from build123d import *

# Parameters (mm, degrees)
F1_ANGLE_BACK  = 30
F1_ANGLE       = 120
F2_R           = 2
F4_DEPTH       = 25
F4_DEPTH_BACK  = 25
F5_DEPTH       = 25
F5_DEPTH_BACK  = 25
F8_R           = 5
F10_DEPTH      = 33.4248144675
F10_DEPTH_BACK = 33.4248144675
F12_DEPTH      = 50
F12_DEPTH_BACK = 50


# Not quite as in the source:
# - after a boolean that leaves OpenCascade's solid faulty, fix() repairs it
# - a feature of the source that left no trace in its solid (it failed there, or was rolled back) is left out


with BuildPart() as f1:
    # F0 (on Top) → F1 (revolve)
    with BuildSketch(Plane.XY, mode=Mode.PRIVATE) as f1_sk:
        with BuildLine():
            Line((9.6206148389, -1.9516889929), (7.6821408379, -2.0284350604))
            Line((7.6821408379, -2.0284350604), (30.2427770644, -88.5876107865))
            ThreePointArc((30.2427770644, -88.5876107865), (29.2549191731, -93.4242240292), (24.8238143675, -95.6))
            Line((24.8238143675, -95.6), (-24.8238143675, -95.6))
            ThreePointArc((-24.8238143675, -95.6), (-29.2549191731, -93.4242240292), (-30.2427770644, -88.5876107865))
            Line((-30.2427770644, -88.5876107865), (-7.6821408379, -2.0284350604))
            Line((-7.6821408379, -2.0284350604), (-9.6206148389, -1.9516889929))
            Line((-9.6206148389, -1.9516889929), (-13.35, -1.9516889929))
            Line((-13.35, -1.9516889929), (-13.35, 37))
            Line((-13.35, 37), (-16.35, 37))
            Line((-16.35, 37), (-16.35, -4.9516889929))
            Line((-16.35, -4.9516889929), (-11.5442770978, -4.9516889929))
            Line((-11.5442770978, -4.9516889929), (-33.1457927948, -87.8309737078))
            ThreePointArc((-33.1457927948, -87.8309737078), (-31.6287253189, -95.2586297591), (-24.8238143675, -98.6))
            Line((-24.8238143675, -98.6), (24.8238143675, -98.6))
            ThreePointArc((24.8238143675, -98.6), (31.6287253189, -95.2586297591), (33.1457927948, -87.8309737078))
            Line((33.1457927948, -87.8309737078), (11.5442770978, -4.9516889929))
            Line((11.5442770978, -4.9516889929), (16.35, -4.9516889929))
            Line((16.35, -4.9516889929), (16.35, 37))
            Line((16.35, 37), (13.35, 37))
            Line((13.35, 37), (13.35, -1.9516889929))
            Line((13.35, -1.9516889929), (9.6206148389, -1.9516889929))
        make_face()
    revolve(f1_sk.sketch.rotate(Axis((0.7210588083, 37, 0), (1, 0, 0)), -F1_ANGLE_BACK), axis=Axis((0.7210588083, 37, 0), (1, 0, 0)), revolution_arc=F1_ANGLE)

    # F2
    f2_edges = [f1.edges().sort_by_distance(p)[0] for p in [
        (7.682141, 3.200384, -19.514218),
        (11.544277, 0.668772, -20.975844),
        (16.35, 0.668772, -20.975844),
        (-7.682141, 3.200384, -19.514218),
        (-16.35, 0.668772, -20.975844),
        (-11.544277, 0.668772, -20.975844),
    ]]
    fillet(f2_edges, radius=F2_R)

    # F3 (on Right) → F4 (join, two sides)
    with BuildSketch(Plane.YZ) as f4_sk:
        with BuildLine():
            Line((51.55, 6), (26.6076951546, 6))
            Line((26.6076951546, 6), (34.6184301396, 1.375))
            ThreePointArc((34.6184301396, 1.375), (37.711752374, 2.6562960223), (39.75, 0))
            ThreePointArc((39.75, 0), (38.9445436483, -1.9445436483), (37, -2.75))
            Line((37, -2.75), (37, -6))
            Line((37, -6), (51.55, -6))
            Line((51.55, -6), (51.55, 6))
        make_face()
        with BuildLine():
            ThreePointArc((47.3738633754, 0.95), (47.505593785, 0.4830952573), (47.55, 0))
            ThreePointArc((47.55, 0), (47.505593785, -0.4830952573), (47.3738633754, -0.95))
            ThreePointArc((47.3738633754, -0.95), (46.7738329701, -1.8738329701), (45.85, -2.4738633754))
            ThreePointArc((45.85, -2.4738633754), (44.9, -2.65), (43.95, -2.4738633754))
            ThreePointArc((43.95, -2.4738633754), (43.0261670299, -1.8738329701), (42.4261366246, -0.95))
            ThreePointArc((42.4261366246, -0.95), (42.25, 0), (42.4261366246, 0.95))
            ThreePointArc((42.4261366246, 0.95), (43.0261670299, 1.8738329701), (43.95, 2.4738633754))
            ThreePointArc((43.95, 2.4738633754), (44.9, 2.65), (45.85, 2.4738633754))
            ThreePointArc((45.85, 2.4738633754), (46.7738329701, 1.8738329701), (47.3738633754, 0.95))
        make_face(mode=Mode.SUBTRACT)
        with BuildLine():
            Line((34.6184301396, 1.375), (26.6076951546, 6))
            Line((26.6076951546, 6), (22.45, 6))
            Line((22.45, 6), (22.45, -6))
            Line((22.45, -6), (37, -6))
            Line((37, -6), (37, -2.75))
            ThreePointArc((37, -2.75), (34.6184301396, -1.375), (34.6184301396, 1.375))
        make_face()
        with BuildLine():
            ThreePointArc((31.5738633754, 0.95), (31.705593785, 0.4830952573), (31.75, 0))
            ThreePointArc((31.75, 0), (31.705593785, -0.4830952573), (31.5738633754, -0.95))
            ThreePointArc((31.5738633754, -0.95), (30.9738329701, -1.8738329701), (30.05, -2.4738633754))
            ThreePointArc((30.05, -2.4738633754), (29.1, -2.65), (28.15, -2.4738633754))
            ThreePointArc((28.15, -2.4738633754), (27.2261670299, -1.8738329701), (26.6261366246, -0.95))
            ThreePointArc((26.6261366246, -0.95), (26.45, 0), (26.6261366246, 0.95))
            ThreePointArc((26.6261366246, 0.95), (27.2261670299, 1.8738329701), (28.15, 2.4738633754))
            ThreePointArc((28.15, 2.4738633754), (29.1, 2.65), (30.05, 2.4738633754))
            ThreePointArc((30.05, 2.4738633754), (30.9738329701, 1.8738329701), (31.5738633754, 0.95))
        make_face(mode=Mode.SUBTRACT)
        with BuildLine():
            Line((43.95, 0.95), (43.95, 2.4738633754))
            ThreePointArc((43.95, 2.4738633754), (43.0261670299, 1.8738329701), (42.4261366246, 0.95))
            Line((42.4261366246, 0.95), (43.95, 0.95))
        make_face()
        with BuildLine():
            Line((45.85, 0.95), (47.3738633754, 0.95))
            ThreePointArc((47.3738633754, 0.95), (46.7738329701, 1.8738329701), (45.85, 2.4738633754))
            Line((45.85, 2.4738633754), (45.85, 0.95))
        make_face()
        with BuildLine():
            ThreePointArc((45.85, -2.4738633754), (46.7738329701, -1.8738329701), (47.3738633754, -0.95))
            Line((47.3738633754, -0.95), (45.85, -0.95))
            Line((45.85, -0.95), (45.85, -2.4738633754))
        make_face()
        with BuildLine():
            ThreePointArc((42.4261366246, -0.95), (43.0261670299, -1.8738329701), (43.95, -2.4738633754))
            Line((43.95, -2.4738633754), (43.95, -0.95))
            Line((43.95, -0.95), (42.4261366246, -0.95))
        make_face()
        with BuildLine():
            Line((30.05, 0.95), (31.5738633754, 0.95))
            ThreePointArc((31.5738633754, 0.95), (30.9738329701, 1.8738329701), (30.05, 2.4738633754))
            Line((30.05, 2.4738633754), (30.05, 0.95))
        make_face()
        with BuildLine():
            Line((28.15, 0.95), (28.15, 2.4738633754))
            ThreePointArc((28.15, 2.4738633754), (27.2261670299, 1.8738329701), (26.6261366246, 0.95))
            Line((26.6261366246, 0.95), (28.15, 0.95))
        make_face()
        with BuildLine():
            ThreePointArc((26.6261366246, -0.95), (27.2261670299, -1.8738329701), (28.15, -2.4738633754))
            Line((28.15, -2.4738633754), (28.15, -0.95))
            Line((28.15, -0.95), (26.6261366246, -0.95))
        make_face()
        with BuildLine():
            ThreePointArc((30.05, -2.4738633754), (30.9738329701, -1.8738329701), (31.5738633754, -0.95))
            Line((31.5738633754, -0.95), (30.05, -0.95))
            Line((30.05, -0.95), (30.05, -2.4738633754))
        make_face()
    extrude(amount=F4_DEPTH)
    extrude(f4_sk.sketch, amount=-F4_DEPTH_BACK)

    # F3 (on Right) → F5 (cut, two sides)
    with BuildSketch(Plane.YZ) as f5_sk:
        with BuildLine():
            Line((37, 0), (34.6184301396, 1.375))
            ThreePointArc((34.6184301396, 1.375), (34.6184301396, -1.375), (37, -2.75))
            Line((37, -2.75), (37, 0))
        make_face()
        with BuildLine():
            ThreePointArc((31.5738633754, -0.95), (31.705593785, -0.4830952573), (31.75, 0))
            ThreePointArc((31.75, 0), (31.705593785, 0.4830952573), (31.5738633754, 0.95))
            Line((31.5738633754, 0.95), (30.05, 0.95))
            Line((30.05, 0.95), (30.05, 2.4738633754))
            ThreePointArc((30.05, 2.4738633754), (29.1, 2.65), (28.15, 2.4738633754))
            Line((28.15, 2.4738633754), (28.15, 0.95))
            Line((28.15, 0.95), (26.6261366246, 0.95))
            ThreePointArc((26.6261366246, 0.95), (26.45, 0), (26.6261366246, -0.95))
            Line((26.6261366246, -0.95), (28.15, -0.95))
            Line((28.15, -0.95), (28.15, -2.4738633754))
            ThreePointArc((28.15, -2.4738633754), (29.1, -2.65), (30.05, -2.4738633754))
            Line((30.05, -2.4738633754), (30.05, -0.95))
            Line((30.05, -0.95), (31.5738633754, -0.95))
        make_face()
    extrude(amount=-F5_DEPTH, mode=Mode.SUBTRACT)
    extrude(f5_sk.sketch, amount=F5_DEPTH_BACK, mode=Mode.SUBTRACT)

    add(f1.part.fix(), mode=Mode.REPLACE)

    # F8
    f8_edges = [f1.edges().sort_by_distance(p)[0] for p in [
        (-20.675, 22.45, -6),
        (-20.675, 22.45, 6),
        (0, 51.55, 6),
        (0, 51.55, -6),
    ]]
    fillet(f8_edges, radius=F8_R)

    # F9 (on Right) → F10 (cut, two sides)
    with BuildSketch(Plane.YZ) as f10_sk:
        Polygon((-115.0443181396, -6), (27.45, -6), (46.55, -6), (89.7687226534, -48.6618503928), (83.2566171885, 31.4302965999), (-50.0242002308, 71.4145377278), (-90.0084450841, 71.4145377278), align=None)
    extrude(amount=F10_DEPTH, mode=Mode.SUBTRACT)
    extrude(f10_sk.sketch, amount=-F10_DEPTH_BACK, mode=Mode.SUBTRACT)

    # F11 (on Right) → F12 (cut, two sides)
    with BuildSketch(Plane.YZ) as f12_sk:
        Polygon((57.0278279483, 8.6879674345), (37, -6), (-77.3825557827, -120.3825557827), (-35.5902947485, -136.9153559208), (64.6576955914, -143.4855163097), (76.9502595067, -111.2705171108), (76.9502595067, -24.7986763716), align=None)
    extrude(amount=-F12_DEPTH, mode=Mode.SUBTRACT)
    extrude(f12_sk.sketch, amount=F12_DEPTH_BACK, mode=Mode.SUBTRACT)


solid = f1.part
The model under review builds one solid part; all positions refer to its coordinate system, in mm. A direction names the side the tool comes from. Coordinates: 2 decimals unless noted, no trailing zeros. Write each loop counter-clockwise with the first axis right and the second up, starting at its lowest first coordinate (ties: lowest second). Pieces come first, ordered by that corner, then holes. Notation, with made-up numbers: (10.5, 16.25) - (36.5, 16.25) arc R13 cw to (36.5, 40.25) - close; hole circle Ø3 at (-5, 7). An arc over 180 degrees is marked (long way). Answer as a JSON object with one key per item and string values. Group by question number.
1. To check wall thickness, follow probe 1 along X at (y, z) = (-61.5, -36); probe 2 along X at (y, z) = (-58, -50); probe 3 along Y at (x, z) = (-10, -92.5). State the ranges of each line that lie inside material, in increasing order.
2. Mouldability with a two-part tool opening along Y and no side actions: class faces 5 (the face through (13.35, 17, -14)), 6 (the face through (0.348, -86.533, -55.919)), 7 (the face through (11.778, 3.186, -19.335)), 8 (the face through (19.43, -38.29, -37.49)) as pulls with the +Y half, pulls with the -Y half, needs draft (parallel to the pull), parting line crosses it, or undercut.
3. Add section A-A (x = 23). Give the boundary of the cut face in (y, z), plus the area to 3 significant figures.
4. Clearance check with flat-ended pins moving along their axes: pin 1 Ø4 at (x, z) = (15, -77.5) entering from +Y (3 decimals); pin 2 Ø12 at (y, z) = (24.5, -24) entering from -X; pin 3 Ø4 at (x, y) = (9, 14) entering from +Z; pin 4 Ø7.5 at (y, z) = (25, -24.5) entering from +X. State where each tip first meets the part, or that it passes through.
5. Machinability: for faces 1 (the face through (-11.822, 3.186, -19.335)), 2 (the face through (-19.125, -37.239, -36.965)), 3 (the face through (16.35, 14, -13)), 4 (the face through (-16.35, 17, -14)), which of the approach directions +Z, -Z, +X, -X, +Y, -Y give a long, thin tool a straight path to every point of the face, cutting with its end or side? Answer none if there is none.
6. Add section B-B (x = 6). Give the boundary of the cut face in (y, z).
Findings:
{
 "1": {"probe 1": "-27.94 to -24.84, 24.84 to 27.94", "probe 2": "-28.59 to -25.49, 25.49 to 28.59", "probe 3": "-62.15 to -58.01"},
 "2": {"face 5": "needs draft", "face 6": "pulls with the -Y half", "face 7": "pulls with the +Y half", "face 8": "undercut"},
 "3": {"outline": "(-98.47, -6) arc R135.6 ccw to (-55.84, -98.84) - (-53.71, -96.71) arc R132.6 cw to (-95.46, -6) - close; (-60.61, -6) arc R97.8 ccw to (-29.09, -72.09) - (-20.67, -63.67) arc R85.9 cw to (-48.69, -6) - close", "area": "1,150 mm²"},
 "4": {"pin 1": "y = -69.125", "pin 2": "x = -16.35", "pin 3": "z = -30.07", "pin 4": "through"},
 "5": {"face 1": "+Z, +Y", "face 2": "none", "face 3": "+Z, -Z, +X, +Y", "face 4": "+Z, -Z, -X, +Y"},
 "6": {"outline": "(-98.47, -6) arc R135.6 ccw to (-55.84, -98.84) - (-53.71, -96.71) arc R132.6 cw to (-95.46, -6) - close"}
}
